Source: CAD feature listing. Evaluate the final solid. Frame: model axes, mm. Face numbers are marked on the shaded views. A direction names the side the tool comes from. Round coordinates to 2 decimals unless told otherwise and drop trailing zeros. Write each loop counter-clockwise with the first axis right and the second up, starting at its lowest first coordinate (ties: lowest second). Pieces come first, ordered by that corner, then holes.
```python
from build123d import *

# Parameters (mm, degrees)
SKETCH1_R           = 2.625
BOSS_EXTRUDE1_DEPTH = 2
SKETCH2_R           = 1.5
BOSS_EXTRUDE2_DEPTH = 5
FILLET1_SIZE        = 3
FILLET1_SIZE_2      = 1.5
SKETCH4_W           = 1
SKETCH4_H           = 1
CUT_EXTRUDE1_DEPTH  = 1


# Read off the part's stored shape, not the designer's step: M3x0.5 Machine Threads Stud1
with BuildPart() as part:
    # Sketch1 → Boss-Extrude1 (new body)
    with BuildSketch(Plane(origin=(0, 0, 0), x_dir=(1, 0, 0), z_dir=(0, 1, 0))):
        with Locations(Location((0, 0, 0), (0, 0, 270))):
            Circle(SKETCH1_R)
    extrude(amount=-BOSS_EXTRUDE1_DEPTH)

    # Sketch2 → Boss-Extrude2 (add)
    with BuildSketch(Plane(origin=(0, -2, 0), x_dir=(-1, 0, 0), z_dir=(0, -1, 0))):
        with Locations(Location((0, 0, 0), (0, 0, 90))):
            Circle(SKETCH2_R)
    extrude(amount=BOSS_EXTRUDE2_DEPTH)

    # M3x0.5 Machine Threads Stud1 outline → M3x0.5 Machine Threads Stud1 (revolve, cut)
    with BuildSketch(Plane.XY):
        Polygon((1.5, -6.7195), (1.2195, -7), (1.5, -7), align=None)
    revolve(axis=Axis((0, 0, 0), (0, 1, 0)), mode=Mode.SUBTRACT)

    # Fillet1
    # an asymmetric fillet: 3, 1.5 mm, written as the material it takes off along each edge
    with BuildSketch(Plane(origin=(0, 0, 0), x_dir=(0, 0, 1), z_dir=(-1, 0, 0))) as fillet1_piece_1:
        with BuildLine():
            Bezier((2.625, -FILLET1_SIZE), (2.625, 0), (2.625 - FILLET1_SIZE_2, 0), weights=[1, 0.707106781, 1])
            Line((2.625 - FILLET1_SIZE_2, 0), (2.625, 0))
            Line((2.625, 0), (2.625, -FILLET1_SIZE))
        make_face()
    revolve(axis=Axis((0, 0, 0), (0, 1, 0)), mode=Mode.SUBTRACT)

    # Sketch4 → Cut-Extrude1 (cut)
    with BuildSketch(Plane(origin=(0, 0, 0), x_dir=(-1, 0, 0), z_dir=(0, 1, 0))):
        with BuildLine():
            Line((-3, 0.5), (-3, -0.5))
            Line((-3, -0.5), (-1.007782219, -0.5))
            ThreePointArc((-1.007782219, -0.5), (-1.125, 0), (-1.007782219, 0.5))
            Line((-1.007782219, 0.5), (-3, 0.5))
        make_face()
        with BuildLine():
            ThreePointArc((-1.007782219, 0.5), (-1.125, 0), (-1.007782219, -0.5))
            Line((-1.007782219, -0.5), (-0.5, -0.5))
            Line((-0.5, -0.5), (-0.5, 0.5))
            Line((-0.5, 0.5), (-1.007782219, 0.5))
        make_face()
        Rectangle(SKETCH4_W, SKETCH4_H)
        with BuildLine():
            Line((0.5, -0.5), (-0.5, -0.5))
            Line((-0.5, -0.5), (-0.5, -1.007782219))
            ThreePointArc((-0.5, -1.007782219), (0, -1.125), (0.5, -1.007782219))
            Line((0.5, -1.007782219), (0.5, -0.5))
        make_face()
        with BuildLine():
            ThreePointArc((0.5, -1.007782219), (0, -1.125), (-0.5, -1.007782219))
            Line((-0.5, -1.007782219), (-0.5, -3))
            Line((-0.5, -3), (0.5, -3))
            Line((0.5, -3), (0.5, -1.007782219))
        make_face()
        with BuildLine():
            Line((0.5, 0.5), (0.5, -0.5))
            Line((0.5, -0.5), (1.007782219, -0.5))
            ThreePointArc((1.007782219, -0.5), (1.09530361, -0.256778118), (1.125, 0))
            ThreePointArc((1.125, 0), (1.09530361, 0.256778118), (1.007782219, 0.5))
            Line((1.007782219, 0.5), (0.5, 0.5))
        make_face()
        with BuildLine():
            ThreePointArc((1.125, 0), (1.09530361, -0.256778118), (1.007782219, -0.5))
            Line((1.007782219, -0.5), (3, -0.5))
            Line((3, -0.5), (3, 0.5))
            Line((3, 0.5), (1.007782219, 0.5))
            ThreePointArc((1.007782219, 0.5), (1.09530361, 0.256778118), (1.125, 0))
        make_face()
        with BuildLine():
            Line((-0.5, 1.007782219), (-0.5, 0.5))
            Line((-0.5, 0.5), (0.5, 0.5))
            Line((0.5, 0.5), (0.5, 1.007782219))
            ThreePointArc((0.5, 1.007782219), (0, 1.125), (-0.5, 1.007782219))
        make_face()
        with BuildLine():
            Line((-0.5, 3), (-0.5, 1.007782219))
            ThreePointArc((-0.5, 1.007782219), (0, 1.125), (0.5, 1.007782219))
            Line((0.5, 1.007782219), (0.5, 3))
            Line((0.5, 3), (-0.5, 3))
        make_face()
    extrude(amount=-CUT_EXTRUDE1_DEPTH, mode=Mode.SUBTRACT)


solid = part.part
```
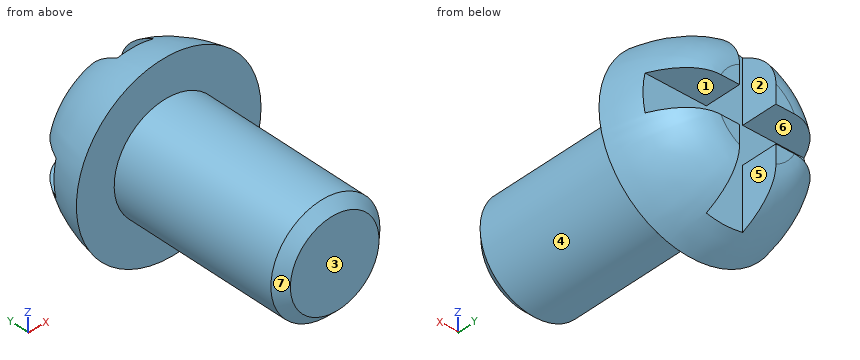
Q1. Section query A-A, the plane y = -3.75. Output: boundary loops of the cut face in (x, z).
Q2. Line query: line 1 (Y direction, x = 0.45, z = 0.3); line 2 (Z direction, x = -1, y = -0.5); line 3 (X direction, y = -3.75, z = 0). Output: solid intervals per line, ascending.
Q3. Pin query (flat end, axial travel): P1, Ø0.5, axis at x = -1.5, y = -0.5, coming from the +Z side; P2, Ø0.5, axis at x = 1, y = -0.5, coming from the -Z side; P3, Ø0.5, axis at x = -1.5, y = -0.5, coming from the -Z side. Return the tip coordinate at first contact, or that it passes through.
Q4. Set-up query: the marked faces 1, 2, 3 and 4. Return all of +Z, -Z, +X, -X, +Y, -Y with unobstructed straight access to the full face (end or side cutting, diameter ignored); none if empty.
Q5. Mould query, pull axis X, two halves, no side actions, for the marked faces 5, 6 and 7. Classes: pulls with the +X half, pulls with the -X half, needs draft (parallel to the pull), parting line crosses it, or undercut.
Filled in:
1. outline: circle Ø3 at (0, 0)
2. line 1: y = -7 to -1
2. line 2: z = -1.68 to -0.5, 0.5 to 1.68
2. line 3: x = -1.5 to 1.5
3. P1: stops at z = 1.6
3. P2: stops at z = -1.91
3. P3: stops at z = -1.6
4. face 1: +X, -X, +Y
4. face 2: +Z, -Z, +Y
4. face 3: +Z, -Z, +X, -X, -Y
4. face 4: -Y
5. face 5: undercut
5. face 6: needs draft
5. face 7: parting line crosses it
